from build123d import *

# Parameters (mm, degrees)
F0_R     = 33.6400886769
F0_R_2   = 24.263041798
F1_DEPTH = 73.4
F2_R     = 5


# Not quite as in the source:
# - a fillet or chamfer that OpenCascade refuses, or shapes differently, is made with other operations: its cross-section is extruded or revolved along the edge and cut away or added


with BuildPart() as f1:
    # F0 (on Front) → F1 (new body)
    with BuildSketch(Plane.XZ):
        with Locations((-20.8813920617, 29.2152203619)):
            Circle(F0_R)
        with Locations((-20.8813920617, 29.2152203619)):
            Circle(F0_R_2, mode=Mode.SUBTRACT)
    extrude(amount=F1_DEPTH)

    # F2
    f2_edges = [f1.edges().sort_by_distance(p)[0] for p in [
        (-54.521481, -73.4, 29.21522),
    ]]
    fillet(f2_edges, radius=F2_R)

    # F3: fillet of radius 5 on 1 edges, made by hand

    # F3_s1 → F3_t2 (revolve, cut)
    with BuildSketch(Plane.XY.offset(29.2152203619)):
        with BuildLine():
            ThreePointArc((7.7586467113, -73.4003968748), (4.6319918458, -71.7466536397), (3.3812497363, -68.4381069026))
            Line((3.3812497363, -68.4381069026), (2.8811131677, -68.4381069026))
            ThreePointArc((2.8811131677, -68.4381069026), (2.8815131677, -70.9190534513), (2.8815131677, -73.4))
            Line((2.8815131677, -73.4), (3.3816497363, -73.9001365685))
            ThreePointArc((3.3816497363, -73.9001365685), (5.5701482238, -73.9001365685), (7.6962498403, -73.896625872))
            Line((7.6962498403, -73.896625872), (7.7586467113, -73.4003968748))
        make_face()
    revolve(axis=Axis((-20.8813920617, -73.4, 29.2152203619), (0, -1, 0)), mode=Mode.SUBTRACT)


solid = f1.part
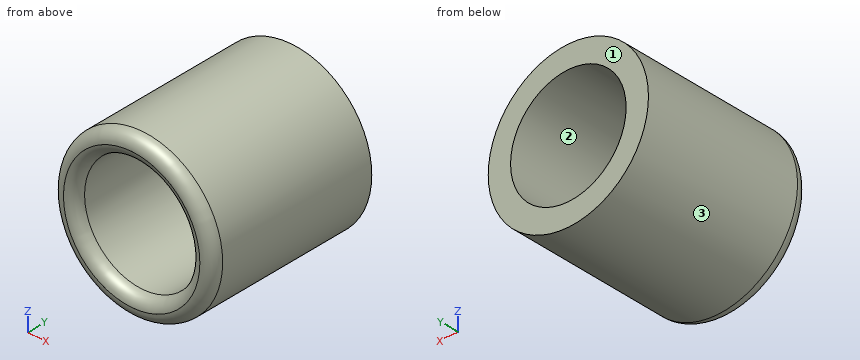
Build history of the part. All positions in model axes, mm. Face numbers are marked on the shaded views. Give positions to 0.01 mm unless a question says otherwise; leave off trailing zeros. Order: outer loops, then holes, each group sorted by start corner. A loop starts at its lowest first (then second) coordinate and runs counter-clockwise, first axis right, second up. Notation, with made-up numbers: M -22,87 L 2,87 A18 ccw 2,96 Z; hole C -20,72.25 d6. An arc over 180 degrees is marked long. Use one line per item in the form item = value.
1) Drop flat-ended pins along their axis: pin 1 (12 mm diameter, centred on y = -23.5, z = 23, fed in from +X); pin 2 (1 mm diameter, centred on x = -44, y = -25, fed in from -Z); pin 3 (8 mm diameter, centred on y = -18, z = 3.5, fed in from -X). Give the stop position or say it passes through.
Calculated:
pin_1 = 12.76
pin_2 = 4.31
pin_3 = -46.57
2) Probe probe 1 along X at (y, z) = (-37, 11); probe 2 along X at (y, z) = (-25.5, 49.5); probe 3 along Z at (x, y) = (-1, -44.5). List the from-to ranges inside material, lowest first.
Calculated:
probe_1 = -49.16 to -36.91, -4.85 to 7.4
probe_2 = -47.72 to -34.19, -7.57 to 5.95
probe_3 = 2.08 to 15.31, 43.12 to 56.35
3) Saw through at A-A (y = -7.5). Give the cut face in (x, z).
Calculated:
outline = C -20.88,29.22 d67.28; hole C -20.88,29.22 d48.53
4) Two-plate mould, pull along X, no slides. Class the marked faces 1, 2 and 3: released by +X, released by -X, zero draft, split by the parting line, or undercut.
Calculated:
face_1 = zero draft
face_2 = undercut
face_3 = split by the parting line
